Geometry: see drawing. Coordinates: mm, zero at the bounding-box minimum. A direction names the side the tool comes from. Coordinates: 2 decimals unless noted, no trailing zeros. Loops run counter-clockwise (first coordinate to the right, second up) from the corner with the lowest first, then second, coordinate; pieces in that order, holes last. Notation, with made-up numbers: M 6.5,78.5 L 32.5,78.5 A15 ccw 32.5,98.5 Z; hole C 69,71.25 d9. An arc over 180 degrees is marked long. One line per question, with ' | ' between items. Start each with the question number.
1. Section query C-C, the plane x = 5. Output: boundary loops of the cut face in (y, z), and give its area (3 significant figures).
2. Section query A-A, the plane y = 67. Output: boundary loops of the cut face in (x, z), and give its area (3 significant figures).
3. Access query for the marked faces 1, 2 and 3. Directions: +Z, -Z, +X, -X, +Y, -Y. A direction counts if a zero-diameter tool reaches every point of the face in a straight line with its end or side. Return the directions, or none.
4. Pin query (flat end, axial travel): P1, Ø1, axis at x = 27.5, y = 13.5, coming from the -Z side; P2, Ø3, axis at x = 11, y = 19.5, coming from the +Z side; P3, Ø2, axis at x = 29.08, y = 29.84, coming from the +Z side; P4, Ø6, axis at y = 71.5, z = 9, coming from the -X side. Return the tip coordinate at first contact, or that it passes through.
5. Ray query, probe 1 along Y at (x, z) = (30.5, 2.25); probe 2 along X at (y, z) = (62, 3); probe 3 along Y at (x, z) = (29, 9.75) (1 decimal). Return the intervals inside material, ascending.
6. Section query B-B, the plane z = 6.5. Output: boundary loops of the cut face in (x, y), and give its area (3 significant figures).
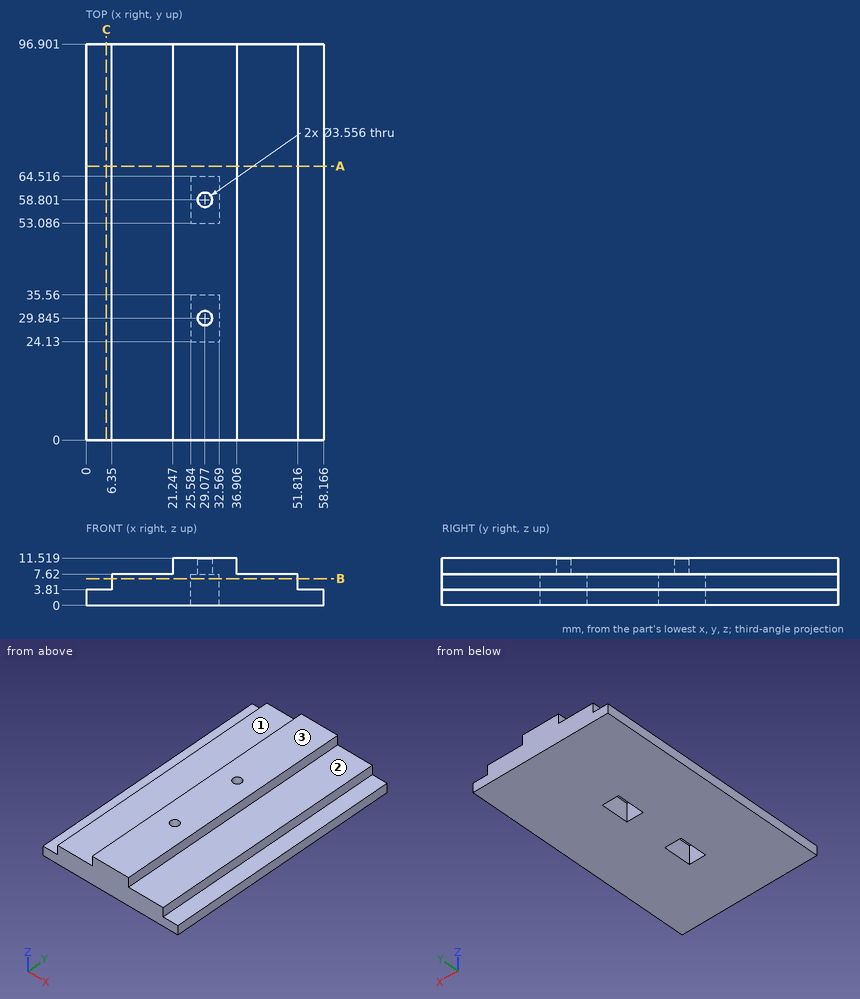
Taken from the geometry:
1) outline: M 0,0 L 96.9,0 L 96.9,3.81 L 0,3.81 Z | area: 369 mm^2
2) outline: M 0,0 L 58.17,0 L 58.17,3.81 L 51.82,3.81 L 51.82,7.62 L 36.91,7.62 L 36.91,11.52 L 21.25,11.52 L 21.25,7.62 L 6.35,7.62 L 6.35,3.81 L 0,3.81 Z | area: 456 mm^2
3) face 1: +Z, -X, +Y, -Y | face 2: +Z, +X, +Y, -Y | face 3: +Z, +X, -X, +Y, -Y
4) P1: z = 0 | P2: z = 7.62 | P3: through | P4: x = 6.35
5) probe 1: 0 to 24.13, 35.56 to 53.09, 64.52 to 96.9 | probe 2: 0 to 25.58, 32.57 to 58.17 | probe 3: 0 to 28.1, 31.6 to 57, 60.6 to 96.9
6) outline: M 6.35,0 L 51.82,0 L 51.82,96.9 L 6.35,96.9 Z; hole M 25.58,24.13 L 32.57,24.13 L 32.57,35.56 L 25.58,35.56 Z; hole M 25.58,53.09 L 32.57,53.09 L 32.57,64.52 L 25.58,64.52 Z | area: 4,250 mm^2
